from build123d import *

# Parameters (mm, degrees)
SALIENTE_EXTRUIR1_DEPTH = 254
CROQUIS2_R              = 7.5
CROQUIS2_R_2            = 22.5
CROQUIS2_R_3            = 1.5
CORTAR_EXTRUIR1_DEPTH   = 254
CROQUIS3_R              = 3
CORTAR_EXTRUIR2_DEPTH   = 292.823782444


with BuildPart() as part:
    # Croquis1 → Saliente-Extruir1 (new body)
    with BuildSketch(Plane.XY):
        Polygon((0, 101.6), (0, 0), (101.6, 0), (101.6, 6.35), (6.35, 6.35), (6.35, 101.6), align=None)
    extrude(amount=SALIENTE_EXTRUIR1_DEPTH)

    # Croquis2 → Cortar-Extruir1 (cut)
    with BuildSketch(Plane.ZY):
        with Locations((101.6, 55)):
            Circle(CROQUIS2_R)
        with BuildLine():
            Line((209.559459459, 77.293611489), (100.586486486, 62.43120383))
            ThreePointArc((100.586486486, 62.43120383), (106.531969619, 60.650281026), (109.1, 55))
            ThreePointArc((109.1, 55), (106.531969619, 49.349718974), (100.586486486, 47.56879617))
            Line((100.586486486, 47.56879617), (209.559459459, 32.706388511))
            ThreePointArc((209.559459459, 32.706388511), (190.1, 55), (209.559459459, 77.293611489))
        make_face()
        with Locations((212.6, 55)):
            Circle(CROQUIS2_R_2)
        with Locations(Location((183.64, 90, 0), (0, 0, 270))):
            Circle(CROQUIS2_R_3)
        with Locations(Location((183.64, 20, 0), (0, 0, 270))):
            Circle(CROQUIS2_R_3)
    extrude(amount=-CORTAR_EXTRUIR1_DEPTH, mode=Mode.SUBTRACT)

    # Croquis3 → Cortar-Extruir2 (cut, through all)
    with BuildSketch(Plane.ZY):
        with Locations(Location((101.6, 79, 0), (0, 0, 270))):
            Circle(CROQUIS3_R)
        with Locations(Location((101.6, 31, 0), (0, 0, 270))):
            Circle(CROQUIS3_R)
    extrude(amount=-CORTAR_EXTRUIR2_DEPTH, mode=Mode.SUBTRACT)


solid = part.part
For this review, take the finished solid that the model builds, in its own axes (mm). A direction names the side the tool comes from. Round coordinates to 2 decimals unless told otherwise and drop trailing zeros. Order: outer loops, then holes, each group sorted by start corner. A loop starts at its lowest first (then second) coordinate and runs counter-clockwise, first axis right, second up. Notation, with made-up numbers: M 18.25,6.5 L 52.25,6.5 A34 ccw 52.25,44.5 Z; hole C 5.25,44.25 d11. An arc over 180 degrees is marked long. Write each question's results on one line, items separated by ' | '. Start each with the question number.
1. To check wall thickness, follow L1, parallel to Z at x = 4.5, y = 20; L2, parallel to Y at x = 89, z = 195.5; L3, parallel to Y at x = 3, z = 101. State the ranges of each line that lie inside material, in increasing order. Write a range as [from, to].
2. Add section D-D (z = 73). State the section outline as (x, y) points, then the cut area to 3 significant figures.
3. Add section B-B (y = 44.5). State the section outline as (x, z) points, then the cut area to 3 significant figures.
4. Add section C-C (x = 52.5). State the section outline as (y, z) points.
5. Clearance check with flat-ended pins moving along their axes: pin 1 Ø6 at (y, z) = (71, 104.5) entering from -X; pin 2 Ø5 at (y, z) = (31, 101.6) entering from +X; pin 3 Ø3 at (y, z) = (84, 216) entering from +X; pin 4 Ø12 at (x, z) = (36.5, 194) entering from +Y. State where each tip first meets the part, or that it passes through.
6. Draft analysis for pull direction Y (two halves, no side actions). For faces 4 (the face through (3.131, 69.966, 155.836)), 5 (the face through (55, 6.35, 125)), 6 (the face through (101.6, 3, 125)), state which applies: pulls with the +Y half, pulls with the -Y half, needs draft (parallel to the pull), parting line crosses it, or undercut.
7. Add section A-A (z = 212.6). State the section outline as (x, y) points, then the cut area to 3 significant figures.
8. Tool access review of faces 1 (the face through (3.13, 40.24, 154.31)), 2 (the face through (0, 40, 125)), 3 (the face through (6.35, 43, 125)): name each direction out of +Z, -Z, +X, -X, +Y, -Y from which nothing blocks a thin tool from reaching the whole face with its end or side.
Output values:
1) L1: [0, 182.14], [185.14, 254] | L2: [0, 6.35] | L3: [0, 28.06], [33.94, 47.51], [62.49, 76.06], [81.94, 101.6]
2) outline: M 0,0 L 101.6,0 L 101.6,6.35 L 6.35,6.35 L 6.35,101.6 L 0,101.6 Z | area: 1,250 mm^2
3) outline: M 0,0 L 6.35,0 L 6.35,123.09 L 0,123.09 Z; M 0,232.5 L 6.35,232.5 L 6.35,254 L 0,254 Z | area: 918 mm^2
4) outline: M 0,0 L 6.35,0 L 6.35,254 L 0,254 Z
5) pin 1: x = 0 | pin 2: through | pin 3: x = 6.35 | pin 4: y = 6.35
6) face 4: undercut | face 5: pulls with the +Y half | face 6: needs draft
7) outline: M 0,0 L 101.6,0 L 101.6,6.35 L 6.35,6.35 L 6.35,32.5 L 0,32.5 Z; M 0,77.5 L 6.35,77.5 L 6.35,101.6 L 0,101.6 Z | area: 964 mm^2
8) face 1: +X, -X | face 2: +Z, -Z, -X, +Y, -Y | face 3: +Z, -Z, +X, +Y
